For this review, take the finished solid that the model builds, in its own axes (mm). A direction names the side the tool comes from. Coordinates: 2 decimals unless noted, no trailing zeros. Loops run counter-clockwise (first coordinate to the right, second up) from the corner with the lowest first, then second, coordinate; pieces in that order, holes last.
```python
from build123d import *

# Parameters (mm, degrees)
BOSS_EXTRUDE1_DEPTH = 49


with BuildPart() as part:
    # Sketch1 → Boss-Extrude1 (new body, symmetric)
    with BuildSketch(Plane.XY):
        with BuildLine():
            Line((-3.6, 3.35), (-3, 0))
            Line((-3, 0), (-2.2, 0))
            Line((-2.2, 0), (-2.735217071, 2.988295315))
            ThreePointArc((-2.735217071, 2.988295315), (-2.659117427, 3.274614514), (-2.390699246, 3.4))
            Line((-2.390699246, 3.4), (-2.2, 3.4))
            Line((-2.2, 3.4), (-2.070472639, 4.88050451))
            ThreePointArc((-2.070472639, 4.88050451), (-1.958261067, 5.108047068), (-1.721804495, 5.2))
            Line((-1.721804495, 5.2), (1.721804495, 5.2))
            ThreePointArc((1.721804495, 5.2), (1.958261067, 5.108047068), (2.070472639, 4.88050451))
            Line((2.070472639, 4.88050451), (2.2, 3.4))
            Line((2.2, 3.4), (2.390699246, 3.4))
            ThreePointArc((2.390699246, 3.4), (2.659117427, 3.274614514), (2.735217071, 2.988295315))
            Line((2.735217071, 2.988295315), (2.2, 0))
            Line((2.2, 0), (3, 0))
            Line((3, 0), (3.6, 3.35))
            ThreePointArc((3.6, 3.35), (3.497487373, 3.597487373), (3.25, 3.7))
            Line((3.25, 3.7), (3, 3.7))
            Line((3, 3.7), (2.835477174, 5.58050451))
            ThreePointArc((2.835477174, 5.58050451), (2.723265602, 5.808047068), (2.486809029, 5.9))
            Line((2.486809029, 5.9), (-2.486809029, 5.9))
            ThreePointArc((-2.486809029, 5.9), (-2.723265602, 5.808047068), (-2.835477174, 5.58050451))
            Line((-2.835477174, 5.58050451), (-3, 3.7))
            Line((-3, 3.7), (-3.25, 3.7))
            ThreePointArc((-3.25, 3.7), (-3.497487373, 3.597487373), (-3.6, 3.35))
        make_face()
    extrude(amount=BOSS_EXTRUDE1_DEPTH, both=True)


solid = part.part
```
Q1. The part is to be moulded in two halves that separate along Y. For faces 1 (the face through (-2.464, 1.473, 0.686)), 2 (the face through (0, 5.4, 49)), 3 (the face through (0, 5.9, 1)), say which applies: +Y half, -Y half, draft (parallel to the pull), parting line (faces both ways), or undercut.
Q2. For pin 1 Ø1.7 at (x, z) = (-0.5, 13.5) entering from -Y, flat-tipped, find the tip position at first contact; note if it passes through.
Q3. Consider section C-C (x = 0.5). State the section outline as (y, z) points.
Q4. Consider section B-B (y = 0.8). State the section outline as (x, z) points.
Q5. Wall thickness on probe 1 along Y at (x, z) = (1, -14); probe 2 along X at (y, z) = (4.55, 17.5); probe 3 along X at (y, z) = (3.5, -23): over which ranges is each line inside the solid? List them lowest first.
Q6. Consider section A-A (z = -27). State the section outline as (x, y) points.
Q7. Machinability: for faces 4 (the face through (0, 5.2, 1)), 5 (the face through (2.471, 1.515, 0.686)), 6 (the face through (-3.304, 1.698, 0.686)), which of the approach directions +Z, -Z, +X, -X, +Y, -Y give a long, thin tool a straight path to every point of the face, cutting with its end or side? Answer none if there is none.
Model answer:
1. face 1: undercut
1. face 2: draft
1. face 3: +Y half
2. pin 1: stops at y = 5.2
3. outline: (5.2, -49) - (5.9, -49) - (5.9, 49) - (5.2, 49) - close
4. outline: (-3.14, -49) - (-2.34, -49) - (-2.34, 49) - (-3.14, 49) - close; (2.34, -49) - (3.14, -49) - (3.14, 49) - (2.34, 49) - close
5. probe 1: y = 5.2 to 5.9
5. probe 2: x = -2.93 to -2.1, 2.1 to 2.93
5. probe 3: x = -3.57 to -2.19, 2.19 to 3.57
6. outline: (-3.6, 3.35) - (-3, 0) - (-2.2, 0) - (-2.74, 2.99) arc R0.35 cw to (-2.39, 3.4) - (-2.2, 3.4) - (-2.07, 4.88) arc R0.35 cw to (-1.72, 5.2) - (1.72, 5.2) arc R0.35 cw to (2.07, 4.88) - (2.2, 3.4) - (2.39, 3.4) arc R0.35 cw to (2.74, 2.99) - (2.2, 0) - (3, 0) - (3.6, 3.35) arc R0.35 ccw to (3.25, 3.7) - (3, 3.7) - (2.84, 5.58) arc R0.35 ccw to (2.49, 5.9) - (-2.49, 5.9) arc R0.35 ccw to (-2.84, 5.58) - (-3, 3.7) - (-3.25, 3.7) arc R0.35 ccw to start
7. face 4: +Z, -Z, -Y
7. face 5: +Z, -Z
7. face 6: +Z, -Z, -X, -Y
